```python
from build123d import *

# Parameters (mm, degrees)
F0_W      = 44
F0_H      = 65
F1_DEPTH  = 11.5
F2_W      = 40
F2_H      = 61
F3_DEPTH  = 10.25
F5_DEPTH  = 11
F6_R      = 1.325
F7_DEPTH  = 7
F10_W     = 15
F10_H     = 6
F11_DEPTH = 6.5
F12_W     = 7
F12_H     = 4.6
F13_DEPTH = 15


with BuildPart() as f1:
    # F0 (on Top) → F1 (new body)
    with BuildSketch(Plane.XY):
        Rectangle(F0_W, F0_H)
    extrude(amount=F1_DEPTH)

    # F2 (on face) → F3 (cut)
    with BuildSketch(Plane.XY.offset(11.5)):
        Rectangle(F2_W, F2_H)
    extrude(amount=-F3_DEPTH, mode=Mode.SUBTRACT)

    # F4 (on face) → F5 (join)
    with BuildSketch(Plane.XY.offset(11.5)):
        with BuildLine():
            Line((20, -30.5), (20, -28.5))
            ThreePointArc((20, -28.5), (18.5857864376, -29.0857864376), (18, -30.5))
            Line((18, -30.5), (20, -30.5))
        make_face()
        with BuildLine():
            ThreePointArc((-18, -30.5), (-18.5857864376, -29.0857864376), (-20, -28.5))
            Line((-20, -28.5), (-20, -30.5))
            Line((-20, -30.5), (-18, -30.5))
        make_face()
        with BuildLine():
            Line((20, 30.5), (18, 30.5))
            ThreePointArc((18, 30.5), (18.5857864376, 29.0857864376), (20, 28.5))
            Line((20, 28.5), (20, 30.5))
        make_face()
        with BuildLine():
            ThreePointArc((-20, 28.5), (-18.5857864376, 29.0857864376), (-18, 30.5))
            Line((-18, 30.5), (-20, 30.5))
            Line((-20, 30.5), (-20, 28.5))
        make_face()
    extrude(amount=-F5_DEPTH)

    # F6 (on face) → F7 (cut)
    with BuildSketch(Plane.XY.offset(11.5)):
        with Locations((-20, -30.5)):
            Circle(F6_R)
        with Locations((-20, 30.5)):
            Circle(F6_R)
        with Locations((20, 30.5)):
            Circle(F6_R)
        with Locations((20, -30.5)):
            Circle(F6_R)
    extrude(amount=-F7_DEPTH, mode=Mode.SUBTRACT)

    # F10 (on face) → F11 (join)
    with BuildSketch(Plane.YZ.offset(22)):
        with Locations((-15, 7.5)):
            Rectangle(F10_W, F10_H)
    extrude(amount=-F11_DEPTH)

    # F12 (on face) → F13 (cut)
    with BuildSketch(Plane(origin=(0, -7.5, 0), x_dir=(-1, 0, 0), z_dir=(0, 1, 0))):
        with Locations((-19.7, 7.5)):
            Rectangle(F12_W, F12_H)
    extrude(amount=-F13_DEPTH, mode=Mode.SUBTRACT)


solid = f1.part
```
Part model, mm, in its own coordinate system. A direction names the side the tool comes from. Round coordinates to 2 decimals unless told otherwise and drop trailing zeros. Order: outer loops, then holes, each group sorted by start corner. A loop starts at its lowest first (then second) coordinate and runs counter-clockwise, first axis right, second up. Notation, with made-up numbers: M 34.25,24 L 82.25,24 A32 cw 82.25,61 Z; hole C -20.5,18 d4. An arc over 180 degrees is marked long. Put each result on its own line as item: value. Start each with the question number.
1. Two-plate mould, pull along X, no slides. Class faces 1 (the face through (19, -15, 9.8)), 2 (the face through (16, -7.5, 8)): +X half, -X half, draft (parallel to the pull), parting line (faces both ways), or undercut.
2. Slice it at D-D on y = 9. List the corners of the cut face in (x, z).
3. Slice it at B-B on z = 2.5. List the corners of the cut face in (x, y).
4. Drill centre lines: probe 1 along X at (y, z) = (4.5, 1.5); probe 2 along X at (y, z) = (-30, 10.5); probe 3 along Y at (x, z) = (-1.5, 1.75). Where is each one in solid material? Low to high. Write a range as [from, to].
5. Slice it at C-C on x = 1. List the corners of the cut face in (y, z).
6. Tool access for faces 3 (the face through (21, -22.5, 8)), 4 (the face through (0, 0, 0)), 5 (the face through (-18.6, 29.07, 6.45)): list every direction of +Z, -Z, +X, -X, +Y, -Y with a clear straight run to the whole face (end or side of a thin tool).
7. Slice it at A-A on y = -20.5. List the corners of the cut face in (x, z).
8. Drop flat-ended pins along their axis: pin 1 (1.5 mm diameter, centred on x = -8.5, y = -3.5, fed in from +Z); pin 2 (2 mm diameter, centred on x = 20, y = -30.5, fed in from +Z); pin 3 (1.3 mm diameter, centred on x = 18.5, y = -17.5, fed in from +Z). Give the stop position or say it passes through.
Findings:
1. face 1: draft
1. face 2: undercut
2. outline: M -22,0 L 22,0 L 22,11.5 L 20,11.5 L 20,1.25 L -20,1.25 L -20,11.5 L -22,11.5 Z
3. outline: M -22,-32.5 L 22,-32.5 L 22,32.5 L -22,32.5 Z; hole M -20,-28.5 A2 cw -18,-30.5 L 18,-30.5 A2 cw 20,-28.5 L 20,28.5 A2 cw 18,30.5 L -18,30.5 A2 cw -20,28.5 Z
4. probe 1: [-22, -20], [20, 22]
4. probe 2: [-22, -21.23], [-18.77, -18.06], [18.06, 18.77], [21.23, 22]
4. probe 3: [-32.5, -30.5], [30.5, 32.5]
5. outline: M -32.5,0 L 32.5,0 L 32.5,11.5 L 30.5,11.5 L 30.5,1.25 L -30.5,1.25 L -30.5,11.5 L -32.5,11.5 Z
6. face 3: +X
6. face 4: -Z, +X, -X, +Y, -Y
6. face 5: +Z
7. outline: M -22,0 L 22,0 L 22,5.2 L 16.2,5.2 L 16.2,9.8 L 22,9.8 L 22,11.5 L 20,11.5 L 20,10.5 L 15.5,10.5 L 15.5,4.5 L 20,4.5 L 20,1.25 L -20,1.25 L -20,11.5 L -22,11.5 Z
8. pin 1: z = 1.25
8. pin 2: z = 4.5
8. pin 3: z = 10.5
